Input: dimensioned drawing with shaded views. Units: mm. Origin: part minimum x, y, z. Coordinates: 2 decimals unless noted, no trailing zeros. Loops run counter-clockwise (first coordinate to the right, second up) from the corner with the lowest first, then second, coordinate; pieces in that order, holes last.
Item 1: Section B-B on x = 4.24. Return loops of the section in (y, z).
Item 2: Section A-A on z = 13.55. Return loops of the section in (x, y), and give its area (3 significant figures).
Item 3: Ray query, line 1 along Z through (x, y) = (4.24, 1.7); line 2 along X through (y, z) = (4.35, 13.5); line 3 along Z through (x, y) = (10.69, 1.45). Return the intervals inside material, ascending.
Item 4: Pull-direction query (Z, two-part tool) for the marked faces 1, 2, 3 and 4; classes: released by +Z, released by -Z, zero draft, split by the parting line, or undercut.
Item 5: Section C-C on y = 4. Return loops of the section in (x, z).
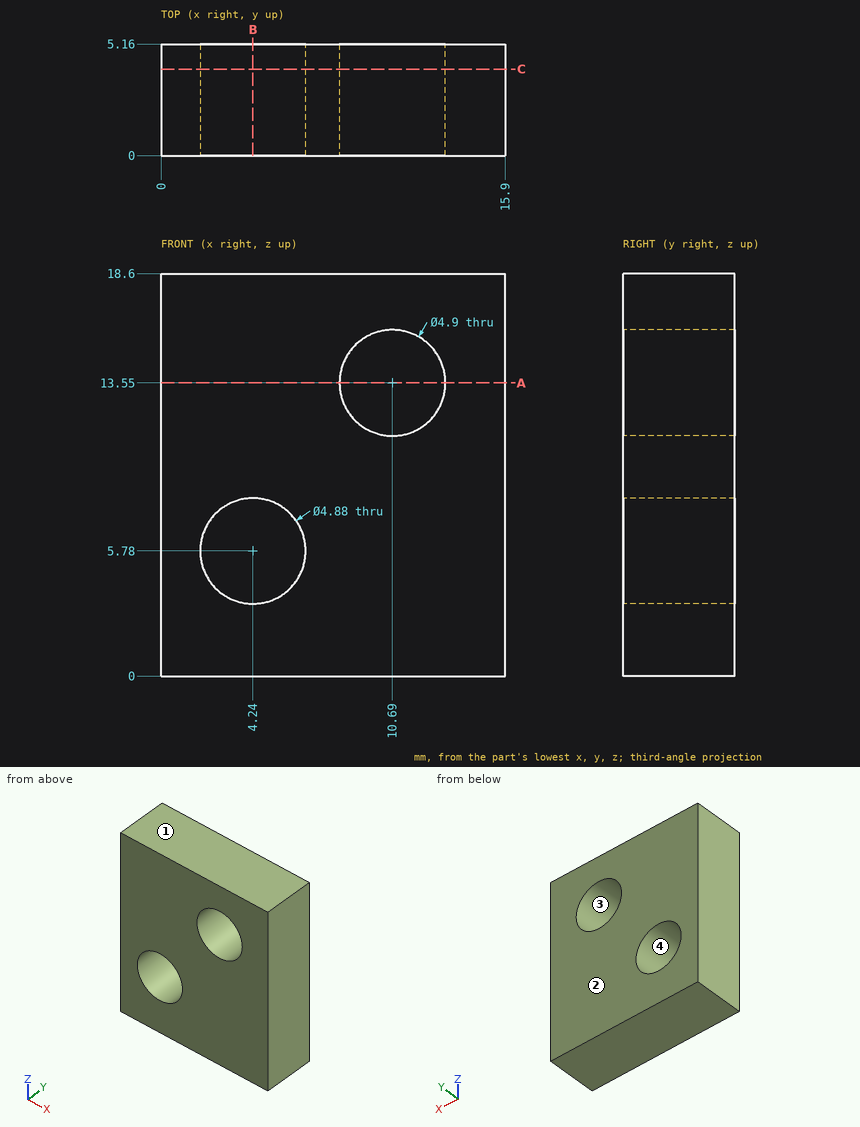
Results found:
1. outline: (0, 0) - (5.16, 0) - (5.16, 3.34) - (0, 3.34) - close; (0, 8.22) - (5.16, 8.22) - (5.16, 18.6) - (0, 18.6) - close
2. outline: (0, 0) - (8.24, 0) - (8.24, 5.16) - (0, 5.16) - close; (13.14, 0) - (15.9, 0) - (15.9, 5.16) - (13.14, 5.16) - close
2. area: 56.8 mm2
3. line 1: z = 0 to 3.34, 8.22 to 18.6
3. line 2: x = 0 to 8.24, 13.14 to 15.9
3. line 3: z = 0 to 11.1, 16 to 18.6
4. face 1: released by +Z
4. face 2: zero draft
4. face 3: undercut
4. face 4: undercut
5. outline: (0, 0) - (15.9, 0) - (15.9, 18.6) - (0, 18.6) - close; hole circle Ø4.88 at (4.24, 5.78); hole circle Ø4.9 at (10.69, 13.55)
